```python
from build123d import *

# Parameters (mm, degrees)
SKETCH1_R           = 7.5
BOSS_EXTRUDE1_DEPTH = 20
BOSS_EXTRUDE2_DEPTH = 5
BOSS_EXTRUDE4_START = 5
BOSS_EXTRUDE4_DEPTH = 5
SCALE1_SCALE        = 0.5


with BuildPart() as part:
    # Sketch1 → Boss-Extrude1 (new body)
    with BuildSketch(Plane(origin=(0, 0, 0), x_dir=(1, 0, 0), z_dir=(0, 1, 0))):
        with Locations(Location((0, 0, 0), (0, 0, 270))):
            Circle(SKETCH1_R)
    extrude(amount=BOSS_EXTRUDE1_DEPTH)

    # Sketch2 → Boss-Extrude2 (add)
    with BuildSketch(Plane(origin=(0, 20, 0), x_dir=(1, 0, 0), z_dir=(0, 1, 0))):
        with BuildLine():
            Line((-3.5, -12.5), (3.5, -12.5))
            ThreePointArc((3.5, -12.5), (9.863961031, -9.863961031), (12.5, -3.5))
            Line((12.5, -3.5), (12.5, 3.5))
            ThreePointArc((12.5, 3.5), (9.863961031, 9.863961031), (3.5, 12.5))
            Line((3.5, 12.5), (-3.5, 12.5))
            ThreePointArc((-3.5, 12.5), (-9.863961031, 9.863961031), (-12.5, 3.5))
            Line((-12.5, 3.5), (-12.5, -3.5))
            ThreePointArc((-12.5, -3.5), (-9.863961031, -9.863961031), (-3.5, -12.5))
        make_face()
    extrude(amount=BOSS_EXTRUDE2_DEPTH)

    # Sketch4 → Boss-Extrude4 (add)
    with BuildSketch(Plane.XZ.offset(BOSS_EXTRUDE4_START)):
        with BuildLine():
            Line((-3.5, 12.5), (3.5, 12.5))
            ThreePointArc((3.5, 12.5), (9.863961031, 9.863961031), (12.5, 3.5))
            Line((12.5, 3.5), (12.5, -3.5))
            ThreePointArc((12.5, -3.5), (9.863961031, -9.863961031), (3.5, -12.5))
            Line((3.5, -12.5), (-3.5, -12.5))
            ThreePointArc((-3.5, -12.5), (-9.863961031, -9.863961031), (-12.5, -3.5))
            Line((-12.5, -3.5), (-12.5, 3.5))
            ThreePointArc((-12.5, 3.5), (-9.863961031, 9.863961031), (-3.5, 12.5))
        make_face()
    extrude(amount=-BOSS_EXTRUDE4_DEPTH)


with BuildPart() as part_1:
    # Scale1: scaled about (0, 10, 0)
    add(part.part.scale(SCALE1_SCALE).moved(Location((0, 5, 0))))


solid = part_1.part
```
Model file for the job. Use its own axes, mm. A direction names the side the tool comes from. Round coordinates to 2 decimals unless told otherwise and drop trailing zeros. Write each loop counter-clockwise with the first axis right and the second up, starting at its lowest first coordinate (ties: lowest second). Pieces come first, ordered by that corner, then holes. Notation, with made-up numbers: (-21.75, 2) -> (12.25, 2) arc R17 ccw to (12.25, 33) -> close; hole circle Ø7 at (23, -31). An arc over 180 degrees is marked (long way). Answer as CSV lines item,"result".
1. Pin check, flat tips, straight feed: pin 1 Ø1.5 at (y, z) = (8.5, 0.5) entering from -X; pin 2 Ø1.5 at (x, y) = (-0.5, 7.5) entering from -Z. Stop position of each tip, or through.
Resolved:
pin 1,"x = -3.75"
pin 2,"z = -3.75"
2. Tool access for faces 1 (the face through (0.165, 9.93, -3.746)), 2 (the face through (0, 2.5, 0)): list every direction of +Z, -Z, +X, -X, +Y, -Y with a clear straight run to the whole face (end or side of a thin tool).
Resolved:
face 1,"none"
face 2,"+Z, -Z, +X, -X, -Y"
3. Slice it at D-D, the plane x = 0. List the corners of the cut face in (y, z), plus the area to 4 significant figures.
Resolved:
outline,"(2.5, -6.25) -> (5, -6.25) -> (5, -3.75) -> (15, -3.75) -> (15, -6.25) -> (17.5, -6.25) -> (17.5, 6.25) -> (15, 6.25) -> (15, 3.75) -> (5, 3.75) -> (5, 6.25) -> (2.5, 6.25) -> close"
area,"137.5 mm²"
4. Slice it at B-B, the plane x = 4.75. List the corners of the cut face in (y, z).
Resolved:
outline,"(2.5, -5.1) -> (5, -5.1) -> (5, 5.1) -> (2.5, 5.1) -> close; (15, -5.1) -> (17.5, -5.1) -> (17.5, 5.1) -> (15, 5.1) -> close"
5. Slice it at C-C, the plane z = 5. List the corners of the cut face in (x, y).
Resolved:
outline,"(-4.86, 2.5) -> (4.86, 2.5) -> (4.86, 5) -> (-4.86, 5) -> close; (-4.86, 15) -> (4.86, 15) -> (4.86, 17.5) -> (-4.86, 17.5) -> close"
6. Drill centre lines: line 1 (Y direction, x = 1.75, z = 4); line 2 (X direction, y = 5.5, z = 0); line 3 (Z direction, x = -2.75, y = 15.25). Where is each one in solid material? Low to high.
Resolved:
line 1,"2.5 to 5, 15 to 17.5"
line 2,"-3.75 to 3.75"
line 3,"-6.14 to 6.14"
7. Slice it at A-A, the plane z = 0. List the corners of the cut face in (x, y).
Resolved:
outline,"(-6.25, 2.5) -> (6.25, 2.5) -> (6.25, 5) -> (3.75, 5) -> (3.75, 15) -> (6.25, 15) -> (6.25, 17.5) -> (-6.25, 17.5) -> (-6.25, 15) -> (-3.75, 15) -> (-3.75, 5) -> (-6.25, 5) -> close"
